Source: CAD feature listing. Evaluate the final solid. Frame: model axes, mm. A direction names the side the tool comes from. Give positions to 0.01 mm unless a question says otherwise; leave off trailing zeros. Order: outer loops, then holes, each group sorted by start corner. A loop starts at its lowest first (then second) coordinate and runs counter-clockwise, first axis right, second up. Notation, with made-up numbers: M -15,21 L -9,21 A18 cw -9,25 Z; hole C -36.75,-33.5 d5. An arc over 180 degrees is marked long. Return JSON: item names as keys, results as strings.
from build123d import *

# Parameters (mm, degrees)
SKETCH1_W           = 50
SKETCH1_H           = 20
BOSS_EXTRUDE1_DEPTH = 1.6
SKETCH2_R           = 0.3
BOSS_EXTRUDE2_DEPTH = 20
SKETCH3_W           = 3.9
SKETCH3_H           = 6
BOSS_EXTRUDE3_DEPTH = 6.95
SKETCH6_R           = 6
BOSS_EXTRUDE4_DEPTH = 8.5
SKETCH7_R           = 4.85
BOSS_EXTRUDE5_DEPTH = 4.5
SKETCH8_R           = 2.5
BOSS_EXTRUDE6_DEPTH = 1.5
CUT_EXTRUDE1_REACH  = 66.004
BOSS_EXTRUDE7_DEPTH = 1.5


with BuildPart() as part:
    # Sketch1 → Boss-Extrude1 (new body)
    with BuildSketch(Plane(origin=(0, 0, 0), x_dir=(1, 0, 0), z_dir=(0, 1, 0))):
        with Locations((25, 10)):
            Rectangle(SKETCH1_W, SKETCH1_H)
    extrude(amount=BOSS_EXTRUDE1_DEPTH)

    # Sketch2 → Boss-Extrude2 (add)
    with BuildSketch(Plane(origin=(0, 1.6, 0), x_dir=(1, 0, 0), z_dir=(0, 1, 0))):
        with Locations(Location((29, 12.54, 0), (0, 0, 90))):
            Circle(SKETCH2_R)
        with Locations(Location((29, 10, 0), (0, 0, 90))):
            Circle(SKETCH2_R)
        with Locations(Location((29, 7.46, 0), (0, 0, 90))):
            Circle(SKETCH2_R)
    extrude(amount=BOSS_EXTRUDE2_DEPTH)

    # Sketch3 → Boss-Extrude3 (add)
    with BuildSketch(Plane(origin=(0, 21.6, 0), x_dir=(1, 0, 0), z_dir=(0, 1, 0))):
        with Locations((28.65, 10)):
            Rectangle(SKETCH3_W, SKETCH3_H)
    extrude(amount=BOSS_EXTRUDE3_DEPTH)

    # Sketch5 → Revolve1 (revolve)
    with BuildSketch(Plane(origin=(0, 25.85, 0), x_dir=(1, 0, 0), z_dir=(0, 1, 0))):
        with BuildLine():
            Line((26.7, 10), (26.7, 12.5))
            ThreePointArc((26.7, 12.5), (25.786983735, 11.395327736), (25.459936306, 10))
            Line((25.459936306, 10), (26.7, 10))
        make_face()
    revolve(axis=Axis((25.459936306, 25.85, -10), (1, 0, 0)))

    # Sketch6 → Boss-Extrude4 (add)
    with BuildSketch(Plane(origin=(0, 1.6, 0), x_dir=(1, 0, 0), z_dir=(0, 1, 0))):
        with Locations(Location((38.5, 10, 0), (0, 0, 90))):
            Circle(SKETCH6_R)
    extrude(amount=BOSS_EXTRUDE4_DEPTH)

    # Sketch7 → Boss-Extrude5 (add)
    with BuildSketch(Plane(origin=(50, 0, 0), x_dir=(0, 0, -1), z_dir=(1, 0, 0))):
        with Locations((10, 1.6)):
            Circle(SKETCH7_R)
    extrude(amount=BOSS_EXTRUDE5_DEPTH)

    # Sketch8 → Boss-Extrude6 (add)
    with BuildSketch(Plane(origin=(0, 1.6, 0), x_dir=(1, 0, 0), z_dir=(0, 1, 0))):
        with Locations(Location((46, 17, 0), (0, 0, 90))):
            Circle(SKETCH8_R)
    boss_extrude6 = extrude(amount=BOSS_EXTRUDE6_DEPTH)

    # Sketch10 → Revolve2 (revolve)
    with BuildSketch(Plane(origin=(46, 0, 0), x_dir=(0, 0, -1), z_dir=(1, 0, 0))):
        with BuildLine():
            Line((19, 3.1), (19, 6.1))
            ThreePointArc((19, 6.1), (18.414213562, 7.514213562), (17, 8.1))
            Line((17, 8.1), (17, 3.1))
            Line((17, 3.1), (19, 3.1))
        make_face()
    revolve2 = revolve(axis=Axis((46, 3.1, -17), (0, 1, 0)))

    # Sketch11 → Cut-Extrude1 (cut, up to next)
    with BuildSketch(Plane(origin=(0, 1.6, 0), x_dir=(1, 0, 0), z_dir=(0, 1, 0)), mode=Mode.PRIVATE) as cut_extrude1_sk1:
        with BuildLine():
            Line((44.5, 19), (47.5, 19))
            ThreePointArc((47.5, 19), (46, 19.5), (44.5, 19))
        make_face()
    cut_extrude1_tool1 = extrude(cut_extrude1_sk1.sketch, amount=CUT_EXTRUDE1_REACH, mode=Mode.PRIVATE) & part.part
    cut_extrude1 = cut_extrude1_tool1.solids().sort_by_distance((46, 1.6, -19.20182))[0]
    add(cut_extrude1, mode=Mode.SUBTRACT)

    # Mirror1: Boss-Extrude6, Revolve2, Cut-Extrude1 across plane
    add(boss_extrude6.mirror(Plane.XY.offset(-10)))
    add(revolve2.mirror(Plane.XY.offset(-10)))
    add(cut_extrude1.mirror(Plane.XY.offset(-10)), mode=Mode.SUBTRACT)

    # Sketch12 → Boss-Extrude7 (add)
    with BuildSketch(Plane.ZY):
        with BuildLine():
            ThreePointArc((-7.5, 1.6), (-9.209430585, 3.971708245), (-12, 3.1))
            Line((-12, 3.1), (-12, 0.1))
            ThreePointArc((-12, 0.1), (-9.209430585, -0.771708245), (-7.5, 1.6))
        make_face()
    extrude(amount=BOSS_EXTRUDE7_DEPTH)

    # Sketch14 → Revolve3 (revolve)
    with BuildSketch(Plane.XY.offset(-10), mode=Mode.PRIVATE) as revolve3_sk:
        with BuildLine():
            Line((-1.5, 3.6), (-4.5, 3.6))
            ThreePointArc((-4.5, 3.6), (-5.914213562, 3.014213562), (-6.5, 1.6))
            Line((-6.5, 1.6), (-1.5, 1.6))
            Line((-1.5, 1.6), (-1.5, 3.6))
        make_face()
    revolve(revolve3_sk.sketch.rotate(Axis((-6.5, 1.6, -10), (1, 0, 0)), 180), axis=Axis((-6.5, 1.6, -10), (1, 0, 0)))


solid = part.part
1. Section query B-B (z = -17). Return loops of the section in (x, y).
Evaluation:
{"outline": "M 0,0 L 50,0 L 50,1.6 L 48.5,1.6 L 48.5,3.1 L 48,3.1 L 48,6.1 A2 ccw 44,6.1 L 44,3.1 L 43.5,3.1 L 43.5,1.6 L 0,1.6 Z"}
2. Draft query along Z for faces 1 (the face through (25, 1, -20)), 2 (the face through (45.9, 2.3, -5.5)), 3 (the face through (50, -1, -10)), 4 (the face through (45, 3.1, -5)). Return one class per face: pulls with the +Z half, pulls with the -Z half, needs draft (parallel to the pull), parting line crosses it, or undercut.
Evaluation:
{"face 1": "pulls with the -Z half", "face 2": "undercut", "face 3": "needs draft", "face 4": "undercut"}
3. Section query A-A (x = 38.5). Return loops of the section in (y, z).
Evaluation:
{"outline": "M 0,-20 L 1.6,-20 L 1.6,-16 L 10.1,-16 L 10.1,-4 L 1.6,-4 L 1.6,0 L 0,0 Z"}
4. Section query D-D (x = 20). Return loops of the section in (y, z), then the cut area to 3 significant figures.
Evaluation:
{"outline": "M 0,-20 L 1.6,-20 L 1.6,0 L 0,0 Z", "area": "32.0 mm^2"}
5. Section query C-C (y = 19). Return loops of the section in (x, z).
Evaluation:
{"outline": "C 29,-12.54 d0.6; C 29,-10 d0.6; C 29,-7.46 d0.6"}
6. Ray query, probe 1 along Y at (x, z) = (3, -18); probe 2 along Y at (x, z) = (39.5, -14.25); probe 3 along X at (y, z) = (3, -3.5). Return the intervals inside material, ascending.
Evaluation:
{"probe 1": "y = 0 to 1.6", "probe 2": "y = 0 to 10.1", "probe 3": "x = 43.55 to 48.45"}
7. Set-up query: faces 5 (the face through (-1, 2, -12)), 6 (the face through (26.7, 23, -9)), 7 (the face through (48, 5, -17)). Return all of +Z, -Z, +X, -X, +Y, -Y with unobstructed straight access to the full face (end or side cutting, diameter ignored); none if empty.
Evaluation:
{"face 5": "-Z, -X, +Y, -Y", "face 6": "-X", "face 7": "+Y"}
8. First-contact query: pin 1 (1 mm diameter, centred on x = 5.5, z = -14.5, fed in from +Y); pin 2 (1.3 mm diameter, centred on y = 0.5, z = -16, fed in from +X); pin 3 (6 mm diameter, centred on x = 32, z = -13.5, fed in from -Y). Flat tips, straight axial feed; report the tip coordinate or a pass-through.
Evaluation:
{"pin 1": "stops at y = 1.6", "pin 2": "stops at x = 50", "pin 3": "stops at y = 0"}
